Verification items for the finished model (mm, model axes). Face numbers are marked on the shaded views. A direction names the side the tool comes from. Coordinates: 2 decimals unless noted, no trailing zeros. Write each loop counter-clockwise with the first axis right and the second up, starting at its lowest first coordinate (ties: lowest second). Pieces come first, ordered by that corner, then holes. Notation, with made-up numbers: (-6.75, 69.25) -> (40.25, 69.25) arc R22 ccw to (40.25, 101.25) -> close; hole circle Ø10 at (-38.5, 36). An arc over 180 degrees is marked (long way). Answer in a Markdown table with one row per item.
```python
from build123d import *

# Parameters (mm, degrees)
F0_R     = 25
F1_DEPTH = 40
F2_W     = 67.128714
F2_H     = 40
F3_DEPTH = 15
F4_R     = 20
F5_DEPTH = 10
F6_R     = 2.5
F7_DEPTH = 50


with BuildPart() as f1:
    # F0 (on Top) → F1 (new body)
    with BuildSketch(Plane.XY):
        Circle(F0_R)
    extrude(amount=F1_DEPTH)

    # F2 (on face) → F3 (cut)
    with BuildSketch(Plane(origin=(0, 0, 0), x_dir=(1, 0, 0), z_dir=(0, 0, -1))):
        Rectangle(F2_W, F2_H)
    extrude(amount=-F3_DEPTH, mode=Mode.SUBTRACT)

    # F4 (on face) → F5 (cut)
    with BuildSketch(Plane(origin=(0, 0, 15), x_dir=(1, 0, 0), z_dir=(0, 0, -1))):
        Circle(F4_R)
    extrude(amount=-F5_DEPTH, mode=Mode.SUBTRACT)

    # F6 (on Front) → F7 (cut, symmetric)
    with BuildSketch(Plane.XZ):
        with Locations((0, 4.646019)):
            Circle(F6_R)
    extrude(amount=F7_DEPTH, both=True, mode=Mode.SUBTRACT)


solid = f1.part
```
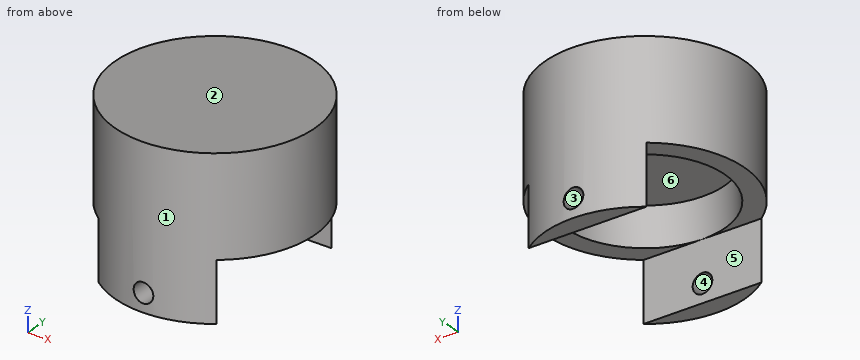
1. Section check B-B, the plane y = 0. Record the boundary of the cut face in (x, z).
Geometry says:
| item | result |
|---|---|
| outline | (-25, 15) -> (-20, 15) -> (-20, 25) -> (20, 25) -> (20, 15) -> (25, 15) -> (25, 40) -> (-25, 40) -> close |
2. Mould release check, pull along X, two halves, no side actions. Record for the marked faces 1, 2 and 3: released by +X, released by -X, zero draft, split by the parting line, or undercut.
Geometry says:
| item | result |
|---|---|
| face 1 | split by the parting line |
| face 2 | zero draft |
| face 3 | undercut |
3. Section check C-C, the plane x = 4.5. Record the boundary of the cut face in (y, z), plus the area to 3 significant figures.
Geometry says:
| item | result |
|---|---|
| outline | (-24.59, 0) -> (-20, 0) -> (-20, 15) -> (-19.49, 15) -> (-19.49, 25) -> (19.49, 25) -> (19.49, 15) -> (20, 15) -> (20, 0) -> (24.59, 0) -> (24.59, 40) -> (-24.59, 40) -> close |
| area | 978 mm^2 |
4. Thickness scan on line 1 (Y direction, x = 0, z = 19.5); line 2 (Z direction, x = 0, y = 21.7). Record the ranges inside material, lowest first. Write a range as from..to.
Geometry says:
| item | result |
|---|---|
| line 1 | -25..-20, 20..25 |
| line 2 | 0..2.15, 7.15..40 |
5. Section check A-A, the plane z = 12.5. Record the boundary of the cut face in (x, y).
Geometry says:
| item | result |
|---|---|
| outline | (-15, -20) arc R25 ccw to (15, -20) -> close; (-15, 20) -> (15, 20) arc R25 ccw to start |
6. Depth check by flat-ended pin: P1, Ø5, axis at x = -11.5, z = 32.5, coming from the -Y side; P2, Ø8, axis at y = -15.5, z = 33.5, coming from the +X side; P3, Ø24, axis at x = 0, y = 0, coming from the -Z side; P4, Ø6, axis at y = -3, z = 34.5, coming from the +X side. Enter the tip coordinate at first touch or a pass-through.
Geometry says:
| item | result |
|---|---|
| P1 | y = -23.32 |
| P2 | x = 22.2 |
| P3 | z = 25 |
| P4 | x = 25 |
7. Tool access check on the marked faces 4, 5 and 6. Record the directions out of +Z, -Z, +X, -X, +Y, -Y that give a thin tool (end or side, any length) a straight path to the whole face; none if there is none.
Geometry says:
| item | result |
|---|---|
| face 4 | +Y, -Y |
| face 5 | -Z, +X, -X |
| face 6 | -Z |
8. Section check D-D, the plane z = 21. Record the boundary of the cut face in (x, y), plus the area to 3 significant figures.
Geometry says:
| item | result |
|---|---|
| outline | circle Ø50 at (0, 0); hole circle Ø40 at (0, 0) |
| area | 707 mm^2 |
